The model under review builds one solid part; all positions refer to its coordinate system, in mm. Face numbers are marked on the shaded views. A direction names the side the tool comes from. Give positions to 0.01 mm unless a question says otherwise; leave off trailing zeros. Loops run counter-clockwise (first coordinate to the right, second up) from the corner with the lowest first, then second, coordinate; pieces in that order, holes last. Notation, with made-up numbers: M 54,78.5 L 66,78.5 A18 cw 66,108.5 Z; hole C -34.5,43 d9. An arc over 180 degrees is marked long. One line per item, written item: value. Start each with the question number.
Q1. We need section A-A on y = -6.35. Write out the cut boundary in (x, z) (3 decimals).
Q2. We need section B-B on y = 68. Write out the cut boundary in (x, z).
Q3. Mouldability with a two-part tool opening along Y and no side actions: class the marked faces 1 and 2 as released by +Y, released by -Y, zero draft, split by the parting line, or undercut.
Q4. To check wall thickness, follow line 1 along X through (y, z) = (-6.35, -4) (3 decimals); line 2 along Y through (x, z) = (4, -1.5); line 3 along Y through (x, z) = (38.5, -5.75). State the ranges of each line that lie inside material, in increasing order. Write a range as from..to.
Q5. For the marked faces 3 and 4, list the 3-axis set-ups (+Z, -Z, +X, -X, +Y, -Y) from which the entire face can be reached by the end or side of a thin tool; tool diameter is ignored.
Q6. For pin 1 (8 mm diameter, centred on x = 84.5, y = 125, fed in from +Z); pin 2 (5 mm diameter, centred on y = 99, z = -2.5, fed in from -X); pin 3 (2 mm diameter, centred on x = -13, y = 29.5, fed in from -Z); pin 4 (5 mm diameter, centred on x = 85.852, y = 123.825, fed in from -Z), all flat-tipped, find the tip position at first contact; note any pin that passes through.
```python
from build123d import *

# Parameters (mm, degrees)
MAIN_BODY_DEPTH          = 6.35
BATTERY_SPACING_DEPTH    = 2.54
SKETCH8_R                = 4.064
LIGHT_SOCKETS_DEPTH      = 12.7
LIGHT_LEADS_POCKET_DEPTH = 6.35
WIRE_TRAIL_DEPTH         = 2.54
LEAD_ROOM_DEPTH          = 7.62
FILLET1_R                = 7.62
TAB_SLOTS_DEPTH          = 1.651
SKETCH14_W               = 12.7
SKETCH14_H               = 6.35
SCREW_MOUNT_DEPTH        = 12.7
CUT_EXTRUDE1_DEPTH       = 179.026641265
CUT_EXTRUDE1_DEPTH_BACK  = 179.026641265
SKETCH15_R               = 3.175


# Sheet-metal steps are written as plain solids
with BuildPart() as part:
    # Sketch1 → Main Body (new body)
    with BuildSketch(Plane.XY):
        Polygon((-53.975, 0), (53.975, 0), (57.15, 82.161327118), (101.6, 101.6), (101.6, 146.05), (-101.6, 146.05), (-101.6, 101.6), (-57.15, 82.161327118), align=None)
    extrude(amount=-MAIN_BODY_DEPTH)

    # Sketch7 → Battery Spacing (cut)
    with BuildSketch(Plane.XY):
        Polygon((-50.564894027, 76.2), (-47.86564661, 6.35), (47.86564661, 6.35), (50.564894027, 76.2), align=None)
    extrude(amount=-BATTERY_SPACING_DEPTH, mode=Mode.SUBTRACT)

    # Sketch8 → Light Sockets (cut)
    with BuildSketch(Plane.XY):
        with Locations((85.852, 123.825)):
            Circle(SKETCH8_R)
        with Locations((-85.852, 123.825)):
            Circle(SKETCH8_R)
        with BuildLine():
            Line((-5.969, 131.318), (5.969, 131.318))
            ThreePointArc((5.969, 131.318), (13.462, 123.825), (5.969, 116.332))
            Line((5.969, 116.332), (-5.969, 116.332))
            ThreePointArc((-5.969, 116.332), (-13.462, 123.825), (-5.969, 131.318))
        make_face()
    extrude(amount=-LIGHT_SOCKETS_DEPTH, mode=Mode.SUBTRACT)

    # Sketch9 → Light Leads Pocket (add)
    with BuildSketch(Plane(origin=(0, 0, -6.35), x_dir=(-1, 0, 0), z_dir=(0, 0, -1))):
        with BuildLine():
            Line((-9.525, 111.765348554), (-9.525, 99.065348554))
            Line((-9.525, 99.065348554), (9.525, 99.065348554))
            Line((9.525, 99.065348554), (9.525, 111.765348554))
            ThreePointArc((9.525, 111.765348554), (18.413001098, 125.621431375), (5.969, 136.398))
            Line((5.969, 136.398), (-5.969, 136.398))
            ThreePointArc((-5.969, 136.398), (-18.413001098, 125.621431375), (-9.525, 111.765348554))
        make_face()
    extrude(amount=LIGHT_LEADS_POCKET_DEPTH)

    # Sketch10 → Wire Trail (cut)
    with BuildSketch(Plane.XY):
        Polygon((-3.175, 116.332), (3.175, 116.332), (3.175, 76.2), (3.175, 6.35), (3.175, 0), (-3.175, 0), align=None)
    extrude(amount=-WIRE_TRAIL_DEPTH, mode=Mode.SUBTRACT)

    # Sketch12 → Lead Room (cut)
    with BuildSketch(Plane.XY.offset(-2.54)):
        with BuildLine():
            Line((-3.175, 116.332), (-5.960094489, 116.332))
            ThreePointArc((-5.960094489, 116.332), (-13.36178344, 123.73368895), (-5.960094489, 131.135377901))
            Line((-5.960094489, 131.135377901), (6.000168296, 131.135377901))
            ThreePointArc((6.000168296, 131.135377901), (13.401857247, 123.73368895), (6.000168296, 116.332))
            Line((6.000168296, 116.332), (3.175, 116.332))
            Line((3.175, 116.332), (3.175, 103.730451358))
            Line((3.175, 103.730451358), (-3.175, 103.730451358))
            Line((-3.175, 103.730451358), (-3.175, 116.332))
        make_face()
    extrude(amount=-LEAD_ROOM_DEPTH, mode=Mode.SUBTRACT)

    # Fillet1
    fillet1_edges = [part.edges().sort_by_distance(p)[0] for p in [
        (0, 103.730451358, -2.54),
    ]]
    fillet(fillet1_edges, radius=FILLET1_R - 0.0001)  # a hair under: the kernel refuses the full size

    # Sketch13 → Tab Slots (cut)
    with BuildSketch(Plane.XY):
        with BuildLine():
            Line((72.263, 146.05), (72.263, 123.825))
            ThreePointArc((72.263, 123.825), (85.852, 110.236), (99.441, 123.825))
            Line((99.441, 123.825), (99.441, 146.05))
            Line((99.441, 146.05), (72.263, 146.05))
        make_face()
    tab_slots = extrude(amount=-TAB_SLOTS_DEPTH, mode=Mode.SUBTRACT)

    # Mirror1: Tab Slots across plane
    add(tab_slots.mirror(Plane(origin=(0, 0, 0), x_dir=(0, 0, 1), z_dir=(1, 0, 0))), mode=Mode.SUBTRACT)

    # Sketch14 → Screw Mount (add)
    with BuildSketch(Plane.XZ):
        with Locations((47.625, -3.175)):
            Rectangle(SKETCH14_W, SKETCH14_H)
    screw_mount = extrude(amount=SCREW_MOUNT_DEPTH)

    # Mirror2: Screw Mount across plane
    add(screw_mount.mirror(Plane(origin=(0, 0, 0), x_dir=(0, 0, 1), z_dir=(1, 0, 0))))

    # Sketch15 → Cut-Extrude1 (cut, two sides: drawn at the far end of the back side and taken through both)
    with BuildSketch(Plane(origin=(0, 0, -6.35), x_dir=(-1, 0, 0), z_dir=(0, 0, -1)).offset(-CUT_EXTRUDE1_DEPTH_BACK)):
        with Locations((47.625, -6.35)):
            Circle(SKETCH15_R)
        with Locations((-47.625, -6.35)):
            Circle(SKETCH15_R)
    extrude(amount=CUT_EXTRUDE1_DEPTH + CUT_EXTRUDE1_DEPTH_BACK, mode=Mode.SUBTRACT)


solid = part.part
```
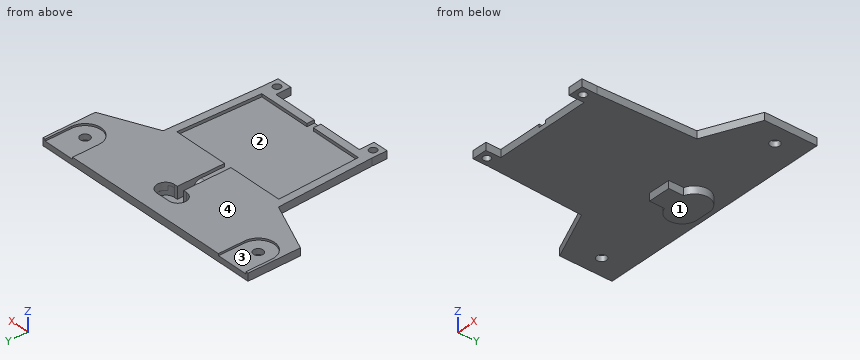
Solved:
1. outline: M -53.975,-6.35 L -50.8,-6.35 L -50.8,0 L -53.975,0 Z; M -44.45,-6.35 L -41.275,-6.35 L -41.275,0 L -44.45,0 Z; M 41.275,-6.35 L 44.45,-6.35 L 44.45,0 L 41.275,0 Z; M 50.8,-6.35 L 53.975,-6.35 L 53.975,0 L 50.8,0 Z
2. outline: M -56.6,-6.35 L 56.6,-6.35 L 56.6,0 L 50.25,0 L 50.25,-2.54 L -50.25,-2.54 L -50.25,0 L -56.6,0 Z
3. face 1: zero draft
3. face 2: undercut
4. line 1: -53.975..-50.8, -44.45..-41.275, 41.275..44.45, 50.8..53.975
4. line 2: 0..6.35, 76.2..116.33, 131.32..146.05
4. line 3: 0..146.05
5. face 3: +Z, +Y
5. face 4: +Z, +X, -X, +Y, -Y
6. pin 1: z = -1.65
6. pin 2: x = -101.37
6. pin 3: z = -6.35
6. pin 4: through
